Read the model definition and answer for the solid it produces. Units are mm, in the model's axes. Round coordinates to 2 decimals unless told otherwise and drop trailing zeros. Order: outer loops, then holes, each group sorted by start corner. A loop starts at its lowest first (then second) coordinate and runs counter-clockwise, first axis right, second up. Notation, with made-up numbers: M 45,67.25 L 95,67.25 A27 ccw 95,85.25 Z; hole C 7.25,70.25 d10. An arc over 180 degrees is marked long. Answer as CSV lines item,"result".
Autodesk Inventor part; units mm, degrees
ref_plane "YZ Plane" through (0, 0, 0) normal (1, 0, 0) x (0, 1, 0)
ref_plane "XZ Plane" through (0, 0, 0) normal (0, 1, 0) x (-1, 0, 0)
ref_plane "XY Plane" through (0, 0, 0) normal (0, 0, 1) x (1, 0, 0)
sketch "Sketch1" plane through (0, 0, 0) normal (0, 1, 0) x (-1, 0, 0)
  line L0 (0, 0) -> (20, 0)
  line L1 (20, 0) -> (20, 20)
  line L2 (20, 20) -> (0, 20)
  line L3 (0, 20) -> (0, 0)
  dimension "d0" = 20
  dimension "d1" = 20
extrude "Extrusion1" add sketch "Sketch1" along normal blind 10
sketch "Sketch2" plane through (0, 10, 0) normal (0, 1, 0) x (1, 0, 0)
  line L0 (0, 0) -> (-20, 0) construction
  line L1 (-10, 0) -> (-10, -20) construction
  line L2 (-20, -20) -> (0, -20) construction
  line L3 (-20, 0) -> (-20, -20) construction
  line L4 (-20, -10) -> (0, -10) construction
  line L5 (0, -20) -> (0, 0) construction
  circle A0 centre (-10, -10) radius 2.5
  dimension "d4" = 5
extrude "Extrusion3" cut sketch "Sketch2" against normal blind 20
properties part number "Insert Test"
Item 1: A cutting plane is placed at A-A, the plane x = -10. Determine the outline of the cut face in (y, z), and give its area (3 significant figures).
Ans:
outline,"M 0,0 L 10,0 L 10,7.5 L 0,7.5 Z; M 0,12.5 L 10,12.5 L 10,20 L 0,20 Z"
area,"150 mm2"
Item 2: Find the intervals of material crossed by probe 1 along X at (y, z) = (6.25, 10); probe 2 along Z at (x, y) = (-10, 4); probe 3 along X at (y, z) = (1.75, 8.5), in increasing order. Write a range as [from, to].
Ans:
probe 1,"[-20, -12.5], [-7.5, 0]"
probe 2,"[0, 7.5], [12.5, 20]"
probe 3,"[-20, -12], [-8, 0]"
Item 3: A cutting plane is placed at C-C, the plane y = 2.75. Determine the outline of the cut face in (x, z).
Ans:
outline,"M -20,0 L 0,0 L 0,20 L -20,20 Z; hole C -10,10 d5"
Item 4: Determine the mould class of faces 1 (the face through (-10.54, 5.07, 12.44)), 2 (the face through (0, 5, 10)), 3 (the face through (-10, 5, 0)), 4 (the face through (-20, 5, 10)) for opening direction X: +X half, -X half, draft (parallel to the pull), parting line (faces both ways), or undercut.
Ans:
face 1,"undercut"
face 2,"+X half"
face 3,"draft"
face 4,"-X half"
Item 5: A cutting plane is placed at B-B, the plane z = 10. Determine the outline of the cut face in (x, y).
Ans:
outline,"M -20,0 L -12.5,0 L -12.5,10 L -20,10 Z; M -7.5,0 L 0,0 L 0,10 L -7.5,10 Z"
